Autodesk Inventor part; units mm, degrees
ref_plane "YZ Plane" through (0, 0, 0) normal (1, 0, 0) x (0, 1, 0)
ref_plane "XZ Plane" through (0, 0, 0) normal (0, 1, 0) x (-1, 0, 0)
ref_plane "XY Plane" through (0, 0, 0) normal (0, 0, 1) x (1, 0, 0)
sketch "Sketch1" plane through (0, 0, 0) normal (0, 0, 1) x (1, 0, 0)
  circle A0 centre (0, 0) radius 0.5
  circle A1 centre (1.4639, -1.3645) radius 0.5
  circle A2 centre (-1.3812, 1.4806) radius 0.5
  circle A3 centre (4.5267, -2.6595) radius 0.5
  circle A4 centre (6.5905, -2.6595) radius 0.5
  circle A5 centre (8.6472, -2.6595) radius 0.5
  line L0 (1.4639, -1.3645) -> (-1.3812, 1.4806) construction
  line L1 (-3.1847, 1.5164) -> (1.4115, -3.0798)
  line L2 (1.4115, -3.0798) -> (3.1792, -1.312)
  line L3 (3.1792, -1.312) -> (-1.417, 3.2842) construction
  line L4 (-1.417, 3.2842) -> (-3.1847, 1.5164)
  arc A6 (3.1792, -1.312) -> (-1.417, 3.2842) centre (-3.8329, -3.728) ccw
  point P0 (0, 0)
  dimension "d0" = 2.5
  dimension "d1" = 6.5
extrude "Extrusion1" add sketch "Sketch1" along normal blind 3.75 contours L4 A6 L2 L1
properties part number "encoder_sensor"
Could you check a few things on this model? Use its own coordinates, in mm. Round coordinates to 2 decimals unless told otherwise and drop trailing zeros. Loops run counter-clockwise (first coordinate to the right, second up) from the corner with the lowest first, then second, coordinate; pieces in that order, holes last. Notation, with made-up numbers: M 44.5,-31.75 L 58.5,-31.75 A10 cw 58.5,-24.75 Z; hole C 88,-6.75 d8. An arc over 180 degrees is marked long. Write item = value, one per line.
1. I want a section at C-C, the plane z = 2.25. Write out the boundary of the cut face in (x, y).
Results below:
outline = M -3.18,1.52 L 1.41,-3.08 L 3.18,-1.31 A7.42 ccw -1.42,3.28 Z; hole C -1.38,1.48 d1; hole C 0,0 d1; hole C 1.46,-1.36 d1
2. I want a section at A-A, the plane y = -1.5. Write out the boundary of the cut face in (x, z).
Results below:
outline = M -0.17,0 L 0.98,0 L 0.98,3.75 L -0.17,3.75 Z; M 1.95,0 L 2.99,0 L 2.99,3.75 L 1.95,3.75 Z
3. Thinking about a two-plate mould opening in X: for faces 1 (the face through (1.356, -0.876, 1.849)), 2 (the face through (-0.92, -0.75, 1.85)), 3 (the face through (-0.108, 0.488, 1.849)), 4 (the face through (1, 0, 3.75)), which applies, +X half, -X half, draft (parallel to the pull), parting line (faces both ways), or undercut?
Results below:
face_1 = undercut
face_2 = -X half
face_3 = undercut
face_4 = draft
4. I want a section at B-B, the plane x = 0.25. Write out the boundary of the cut face in (y, z), and give its area (3 significant figures).
Results below:
outline = M -1.92,0 L -0.43,0 L -0.43,3.75 L -1.92,3.75 Z; M 0.43,0 L 2.46,0 L 2.46,3.75 L 0.43,3.75 Z
area = 13.2 mm²
5. I want a section at D-D, the plane y = 2.75. Write out the boundary of the cut face in (x, z).
Results below:
outline = M -1.95,0 L -0.22,0 L -0.22,3.75 L -1.95,3.75 Z
6. I need wall thicknesses on probe 1 along Y at (x, z) = (0, 1.9); probe 2 along Y at (x, z) = (-1.5, 2.6); probe 3 along X at (y, z) = (-1.5, 3.05). Which ranges of each line are inside material? Lowest first, please.
Results below:
probe_1 = -1.67 to -0.5, 0.5 to 2.62
probe_2 = -0.17 to 0.99, 1.97 to 3.2
probe_3 = -0.17 to 0.98, 1.95 to 2.99
